Can you work these out from the model? Positions are in its coordinate system, mm. A direction names the side the tool comes from. Coordinates: 2 decimals unless noted, no trailing zeros. Write each loop counter-clockwise with the first axis right and the second up, starting at its lowest first coordinate (ties: lowest second). Pieces come first, ordered by that corner, then holes. Notation, with made-up numbers: M -12,-2.75 L 15,-2.75 A8 cw 15,10.25 Z; hole C -12,-34 d3. An arc over 180 degrees is marked long. Use one line per item in the form item = value. Start each with the question number.
```python
from build123d import *

# Parameters (mm, degrees)
F0_W     = 34.221142
F0_H     = 33.016175
F1_DEPTH = 34.798
F2_W     = 16.628581
F2_H     = 16.146597
F3_DEPTH = 32.004
F4_W     = 5.060869
F4_H     = 6.024849
F5_DEPTH = 39.878
F6_R     = 11.215709
F7_DEPTH = 17.018
F8_R     = 5.08


with BuildPart() as f1:
    # F0 (on Front) → F1 (new body)
    with BuildSketch(Plane.XZ):
        with Locations((5.521229, -0.481988)):
            Rectangle(F0_W, F0_H)
    extrude(amount=F1_DEPTH)

    # F2 (on Top) → F3 (join)
    with BuildSketch(Plane.XY):
        with Locations((5.641728, -16.869578)):
            Rectangle(F2_W, F2_H)
    extrude(amount=-F3_DEPTH)

    # F4 (on Top) → F5 (join)
    with BuildSketch(Plane.XY):
        with Locations((5.641728, -17.110572)):
            Rectangle(F4_W, F4_H)
    extrude(amount=-F5_DEPTH)

    # F6 (on face) → F7 (join)
    with BuildSketch(Plane(origin=(0, 0, -39.878), x_dir=(1, 0, 0), z_dir=(0, 0, -1))):
        with Locations((5.309023, 17.110573)):
            Circle(F6_R)
    extrude(amount=F7_DEPTH)

    # F8
    f8_edges = [f1.edges().sort_by_distance(p)[0] for p in [
        (-5.906686, -17.110573, -56.896),
        (-5.906686, -17.110573, -39.878),
    ]]
    fillet(f8_edges, radius=F8_R)


solid = f1.part
```
1) If we mould it in two halves opening along Z, with no side actions, what happens to faces 6 (the face through (5, 0, 0)), 7 (the face through (2, -17, -39.878)), 8 (the face through (6, -8.796, -24)), 9 (the face through (5, -17, 16.026))? For each: +Z half, -Z half, draft (parallel to the pull), parting line (faces both ways), or undercut.
2) Please list where these lines run through material, in increasing order: line 1 (Z direction, x = 8, y = -13); line 2 (Z direction, x = 16.5, y = -21); line 3 (X direction, y = -15.5, z = -26).
3) Will these pins go through, and if not, where does the flat tip stop? pin 1 Ø6 at (x, z) = (4.5, -22) entering from +Y; pin 2 Ø4.5 at (y, z) = (-17.5, -25) entering from +X; pin 3 Ø12 at (y, z) = (-4, -31) entering from -X.
4) Which directions (+Z, -Z, +X, -X, +Y, -Y) give clear straight access to the entire face, cutting with the end or side of a thin tool? Please do faces 1 (the face through (3.111, -17, -36)), 2 (the face through (5.5, -20.3, -32.004)), 3 (the face through (6, -24.943, -24)), 4 (the face through (11.339, -26.568, -48.339)), 5 (the face through (13.956, -17, -24)).
5) Suppose I cut it at C-C on z = -50.5. Please give me the cut outline in (x, y).
6) Suppose I cut it at B-B on z = -36. Please give me the cut outline in (x, y).
7) Suppose I cut it at A-A on x = -8.5. Please give me the cut outline in (y, z), and give its area (3 significant figures).
Computed values:
q1.face_6 = draft
q1.face_7 = undercut
q1.face_8 = undercut
q1.face_9 = +Z half
q2.line_1 = -56.9 to -39.88, -32 to 16.03
q2.line_2 = -16.99 to 16.03
q2.line_3 = -2.67 to 13.96
q3.pin_1 = -8.8
q3.pin_2 = 13.96
q3.pin_3 = -2.67
q4.face_1 = -X, +Y, -Y
q4.face_2 = none
q4.face_3 = +X, -X, -Y
q4.face_4 = -Z
q4.face_5 = +X, +Y, -Y
q5.outline = C 5.31,-17.11 d22.43
q6.outline = M 3.11,-20.12 L 8.17,-20.12 L 8.17,-14.1 L 3.11,-14.1 Z
q7.outline = M -34.8,-16.99 L 0,-16.99 L 0,16.03 L -34.8,16.03 Z
q7.area = 1,150 mm²
